The listing builds one solid part. Answer for the finished solid, in the listing's coordinates (mm). A direction names the side the tool comes from. Give positions to 0.01 mm unless a question says otherwise; leave off trailing zeros. Write each loop counter-clockwise with the first axis right and the second up, starting at its lowest first coordinate (ties: lowest second). Pieces come first, ordered by that corner, then holes. Notation, with made-up numbers: (-24.5, 2) - (-8.5, 2) arc R19 cw to (-8.5, 32) - close; hole circle Ø6 at (87, 80.5). An arc over 180 degrees is marked (long way). Answer as CSV lines item,"result". Start each with the question number.
(1) Each of these flat-tipped pins is pushed along its axis until it touches: pin 1 Ø5 at (x, z) = (-3, -5.5) entering from -Y; pin 2 Ø1.5 at (x, z) = (-34, -13.5) entering from +Y; pin 3 Ø4 at (x, z) = (-39, -30.5) entering from +Y. Where does it stop, or does it pass through?
(2) For a pull along Z with two mould halves and no side action, classify faces 1 (the face through (-33, 1, -7)), 2 (the face through (45, 10, 1)) as pulls with the +Z half, pulls with the -Z half, needs draft (parallel to the pull), parting line crosses it, or undercut.
(3) Find section C-C (x = -21). Write down the section's boundary in (y, z), then the cut area to 3 significant figures.
(4) Straight lines are drawn through the part: probe 1 along Z at (x, y) = (8.5, 11); probe 2 along X at (y, z) = (5.25, -25.5); probe 3 along X at (y, z) = (17, -26). For each, find the intervals that lie inside material, in ascending order.
(5) Find section B-B (z = 24). Write down the section's boundary in (x, y), then the cut area to 3 significant figures.
(6) For faces 3 (the face through (-28, 1, -7)), 4 (the face through (41, 5, -29)), 5 (the face through (33, 17, 35)), 6 (the face through (11.8, 4.5, 24)), 7 (the face through (-32.3, 1.5, 0)), determine the directions among +Z, -Z, +X, -X, +Y, -Y from which every point of the face is accessible in a straight line to the end or side of a thin tool.
(7) Find section D-D (z = 14.5). Write down the section's boundary in (x, y), then the cut area to 3 significant figures.
(8) Find section A-A (y = 16). Write down the section's boundary in (x, z), then the cut area to 3 significant figures.
from build123d import *

# Parameters (mm, degrees)
SKETCH_1_W                  = 90
SKETCH_1_H                  = 72
EXTRUDE_1_DEPTH             = 21
CUT_EXTRUDE_1_DEPTH         = 72
FILLET_1_R                  = 0.5
FILLET_2_R                  = 0.2
CUT_EXTRUDE_2_DEPTH         = 28
SKETCH_6_W                  = 5
SKETCH_6_H                  = 2
CUT_EXTRUDE_3_DEPTH         = 2.4
FILLET_3_R                  = 0.5
EXTRUDE_2_DEPTH             = 3.5
FILLET_4_R                  = 1
FILLET_5_R                  = 0.3
CHAMFER_1_SIZE              = 1
SKETCH_8_W                  = 2.9
SKETCH_8_H                  = 4
EXTRUDE_3_DEPTH             = 2.5
CHAMFER_2_SIZE              = 2
CHAMFER_2_SIZE2             = 1.400415076
FILLET_6_R                  = 0.2
FILLET_7_R                  = 0.3
FILLET_8_R                  = 0.2
SKETCH_9_W                  = 15.2
SKETCH_9_H                  = 5
CUT_EXTRUDE_4_DEPTH         = 36
SKETCH_10_W                 = 7.6
SKETCH_10_H                 = 5
CUT_EXTRUDE_5_DEPTH         = 4
CUT_EXTRUDE_6_DEPTH         = 72
SKETCH_12_W                 = 86
SKETCH_12_H                 = 68
CUT_EXTRUDE_7_DEPTH         = 14.5
SKETCH_13_W                 = 24
SKETCH_13_H                 = 16
CUT_EXTRUDE_8_DEPTH         = 5
MIRROR_4_COPY_1_SKETCH_W    = 24
MIRROR_4_COPY_1_SKETCH_H    = 16
MIRROR_4_COPY_1_DEPTH       = 5
EXTRUDE_4_DEPTH             = 7
MIRROR_6_COPY_1_DEPTH       = 7
SKETCH_15_W                 = 20
SKETCH_15_H                 = 2
EXTRUDE_5_DEPTH             = 2
SKETCH_17_W                 = 4
SKETCH_17_H                 = 2
EXTRUDE_6_DEPTH             = 1
CHAMFER_3_SIZE              = 1
CHAMFER_3_SIZE2             = 1.428148007
CHAMFER_3_OF_MIRROR_8_SIZE2 = 1.428148007
CHAMFER_3_OF_MIRROR_8_SIZE  = 1


with BuildPart() as part:
    # 草图1 → 凸台-拉伸1 (new body)
    with BuildSketch(Plane(origin=(0, 0, 0), x_dir=(1, 0, 0), z_dir=(0, 1, 0))):
        Rectangle(SKETCH_1_W, SKETCH_1_H)
    extrude(amount=EXTRUDE_1_DEPTH)

    # 草图4 → 切除-拉伸1 (cut)
    with BuildSketch(Plane.XY.offset(36)):
        Polygon((14.3, 0), (14.3, 1.5), (15.489963906, 2.965295015), (17.6, 3.5), (17.6, 5), (13.598917425, 4.003578801), (10, 5), (-17.6, 5), (-17.9, 0), align=None)
    extrude(amount=-CUT_EXTRUDE_1_DEPTH, mode=Mode.SUBTRACT)

    # 圆角1
    fillet_1_edges = [part.edges().sort_by_distance(p)[0] for p in [
        (17.6, 5, 0),
        (17.6, 3.5, 0),
    ]]
    fillet(fillet_1_edges, radius=FILLET_1_R)

    # 圆角2
    fillet_2_edges = [part.edges().sort_by_distance(p)[0] for p in [
        (14.3, 0, 0),
        (-17.9, 0, 0),
        (-17.6, 5, 0),
        (15.489963906, 2.965295015, 0),
        (14.3, 1.5, 0),
    ]]
    fillet(fillet_2_edges, radius=FILLET_2_R)

    # 草图5 → 切除-拉伸2 (cut)
    with BuildSketch(Plane.ZY.offset(45)):
        Polygon((5.6, 0), (5.6, 2.4), (7.6, 2.4), (7.6, 5), (-7.6, 5), (-7.6, 2.4), (-5.6, 2.4), (-5.6, 0), align=None)
    extrude(amount=-CUT_EXTRUDE_2_DEPTH, mode=Mode.SUBTRACT)

    # 草图6 → 切除-拉伸3 (cut)
    with BuildSketch(Plane.XZ):
        with Locations((-30.5, 6.6)):
            Rectangle(SKETCH_6_W, SKETCH_6_H)
    cut_extrude_3 = extrude(amount=-CUT_EXTRUDE_3_DEPTH, mode=Mode.SUBTRACT)

    # 镜向1: 切除-拉伸3 across plane
    add(cut_extrude_3.mirror(Plane(origin=(0, 0, 0), x_dir=(1, 0, 0), z_dir=(0, 0, -1))), mode=Mode.SUBTRACT)

    # 圆角3
    fillet_3_edges = [part.edges().sort_by_distance(p)[0] for p in [
        (-31.205820162, 5, -7.6),
        (-31.205820162, 5, 7.6),
    ]]
    fillet(fillet_3_edges, radius=FILLET_3_R)

    # 草图7 → 凸台-拉伸2 (add)
    with BuildSketch(Plane.XZ.offset(-5)):
        Polygon((-33, 3.2), (-33, -3.2), (-28, -3.2), (-32, -1), (-32, 1), (-28, 3.2), align=None)
    extrude(amount=EXTRUDE_2_DEPTH)

    # 圆角4
    fillet_4_edges = [part.edges().sort_by_distance(p)[0] for p in [
        (-32, 3.25, -1),
        (-32, 3.25, 1),
    ]]
    fillet(fillet_4_edges, radius=FILLET_4_R)

    # 圆角5
    fillet_5_edges = [part.edges().sort_by_distance(p)[0] for p in [
        (-28, 3.25, 3.2),
        (-28, 3.25, -3.2),
    ]]
    fillet(fillet_5_edges, radius=FILLET_5_R)

    # 倒角1
    chamfer_1_edges = [part.edges().sort_by_distance(p)[0] for p in [
        (-33, 3.25, 3.2),
        (-33, 3.25, -3.2),
    ]]
    chamfer(chamfer_1_edges, length=CHAMFER_1_SIZE)

    # 草图8 → 凸台-拉伸3 (add)
    with BuildSketch(Plane.XZ.offset(-5)):
        with Locations((-35.91, 0)):
            Rectangle(SKETCH_8_W, SKETCH_8_H)
    extrude(amount=EXTRUDE_3_DEPTH)

    # 倒角2
    chamfer_2_edges = [part.edges().sort_by_distance(p)[0] for p in [
        (-34.46, 2.5, 0),
    ]]
    chamfer_2_side = [part.faces().sort_by_distance(p)[0] for p in [
        (-35.91, 2.5, 0),
    ]]
    chamfer(chamfer_2_edges, length=CHAMFER_2_SIZE, length2=CHAMFER_2_SIZE2, reference=chamfer_2_side[0])

    # 圆角6
    fillet_6_edges = [part.edges().sort_by_distance(p)[0] for p in [
        (-37.36, 5, 0),
        (-37.36, 3.75, 2),
        (-35.91, 5, -2),
        (-37.36, 3.75, -2),
        (-34.46, 5, 0),
        (-35.91, 5, 2),
        (-37.36, 2.5, 0),
        (-36.91, 2.5, -2),
        (-34.46, 4.450207538, -2),
        (-35.46, 3.200207538, -2),
    ]]
    fillet(fillet_6_edges, radius=FILLET_6_R)

    # 圆角7
    # the kernel refuses this fillet: 0.3 mm, written as the material it takes off along each edge
    with BuildSketch(Plane(origin=(-36.554589637, 2.8, -2), x_dir=(0.5735764363510475, -0.8191520442889909, 0), z_dir=(0.8191520442889909, 0.5735764363510475, 0))) as fillet_7_piece_1:
        with BuildLine():
            CenterArc((0.1, -0.2), 0.2, 0, 90)
            Line((0.3, -0.2), (0.3, 0))
            Line((0.3, 0), (0.1, 0))
        make_face()
    revolve(axis=Axis((-36.554589637, 2.8, -2), (0, 0, -1)), revolution_arc=35, mode=Mode.SUBTRACT)
    with BuildSketch(Plane(origin=(-36.46, 2.5, 2.236474092), x_dir=(0.8191520442890007, 0.5735764363510335, 0), z_dir=(0, 0, -1))) as fillet_7_piece_2:
        with BuildLine():
            CenterArc((FILLET_7_R * 0.315298788879, -FILLET_7_R), FILLET_7_R, 90, 35)
            Line((-FILLET_7_R * 0.258277647472, -FILLET_7_R * 0.180847955711), (0, 0))
            Line((0, 0), (FILLET_7_R * 0.315298788879, 0))
        make_face()
    extrude(amount=4.236474092, mode=Mode.SUBTRACT)

    # 圆角8
    fillet_8_edges = [part.edges().sort_by_distance(p)[0] for p in [
        (-34.46, 3.900415076, 0.1),
        (-34.522857251, 3.93313649, -1.945574265),
    ]]
    fillet(fillet_8_edges, radius=FILLET_8_R)

    # 草图9 → 切除-拉伸4 (cut)
    with BuildSketch(Plane(origin=(45, 0, 0), x_dir=(0, 0, -1), z_dir=(1, 0, 0))):
        with Locations((0, 2.5)):
            Rectangle(SKETCH_9_W, SKETCH_9_H)
    extrude(amount=-CUT_EXTRUDE_4_DEPTH, mode=Mode.SUBTRACT)

    # 草图10 → 切除-拉伸5 (cut)
    with BuildSketch(Plane(origin=(0, 0, 7.6), x_dir=(-1, 0, 0), z_dir=(0, 0, -1))):
        with Locations((-13.8, 2.5)):
            Rectangle(SKETCH_10_W, SKETCH_10_H)
    cut_extrude_5 = extrude(amount=-CUT_EXTRUDE_5_DEPTH, mode=Mode.SUBTRACT)

    # 镜向2: 切除-拉伸5 across plane
    add(cut_extrude_5.mirror(Plane(origin=(0, 0, 0), x_dir=(1, 0, 0), z_dir=(0, 0, -1))), mode=Mode.SUBTRACT)

    # 草图11 → 切除-拉伸6 (cut)
    with BuildSketch(Plane.XY.offset(36)):
        Polygon((-37, 21), (37, 21), (28.3, 12.3), (-28.3, 12.3), align=None)
    extrude(amount=-CUT_EXTRUDE_6_DEPTH, mode=Mode.SUBTRACT)

    # 草图12 → 切除-拉伸7 (cut)
    with BuildSketch(Plane(origin=(0, 21, 0), x_dir=(1, 0, 0), z_dir=(0, 1, 0))):
        Rectangle(SKETCH_12_W, SKETCH_12_H)
    extrude(amount=-CUT_EXTRUDE_7_DEPTH, mode=Mode.SUBTRACT)

    # 草图13 → 切除-拉伸8 (cut)
    with BuildSketch(Plane(origin=(0, 6.5, 0), x_dir=(1, 0, 0), z_dir=(0, 1, 0))):
        with Locations((31, -26)):
            Rectangle(SKETCH_13_W, SKETCH_13_H)
    cut_extrude_8 = extrude(amount=-CUT_EXTRUDE_8_DEPTH, mode=Mode.SUBTRACT)

    # 镜向3: 切除-拉伸8 across plane
    add(cut_extrude_8.mirror(Plane(origin=(0, 0, 0), x_dir=(1, 0, 0), z_dir=(0, 0, -1))), mode=Mode.SUBTRACT)

    # 镜向4: 切除-拉伸8 across plane
    add(cut_extrude_8.mirror(Plane.ZY), mode=Mode.SUBTRACT)

    # 镜向4 copy 1 sketch → 镜向4 copy 1 (cut)
    with BuildSketch(Plane(origin=(0, 6.5, 0), x_dir=(-1, 0, 0), z_dir=(0, 1, 0))):
        with Locations((31, -26)):
            Rectangle(MIRROR_4_COPY_1_SKETCH_W, MIRROR_4_COPY_1_SKETCH_H)
    extrude(amount=-MIRROR_4_COPY_1_DEPTH, mode=Mode.SUBTRACT)

    # 草图14 → 凸台-拉伸4 (add)
    with BuildSketch(Plane(origin=(0, 1.5, 0), x_dir=(1, 0, 0), z_dir=(0, 1, 0))):
        Polygon((35, -34), (43, -34), (43, -26), (41, -26), (41, -32), (35, -32), align=None)
    extrude_4 = extrude(amount=EXTRUDE_4_DEPTH)

    # 镜向5: 凸台-拉伸4 across plane
    add(extrude_4.mirror(Plane(origin=(0, 0, 0), x_dir=(1, 0, 0), z_dir=(0, 0, -1))))

    # 镜向6: 凸台-拉伸4 across plane
    add(extrude_4.mirror(Plane.ZY))

    # 镜向6 copy 1 sketch → 镜向6 copy 1 (add)
    with BuildSketch(Plane(origin=(0, 1.5, 0), x_dir=(-1, 0, 0), z_dir=(0, 1, 0))):
        Polygon((35, -34), (43, -34), (43, -26), (41, -26), (41, -32), (35, -32), align=None)
    extrude(amount=MIRROR_6_COPY_1_DEPTH)

    # 草图15 → 凸台-拉伸5 (add)
    with BuildSketch(Plane(origin=(0, 6.5, 0), x_dir=(1, 0, 0), z_dir=(0, 1, 0))):
        with Locations((0, 33)):
            Rectangle(SKETCH_15_W, SKETCH_15_H)
    extrude_5 = extrude(amount=EXTRUDE_5_DEPTH)

    # 镜向7: 凸台-拉伸5 across plane
    add(extrude_5.mirror(Plane(origin=(0, 0, 0), x_dir=(1, 0, 0), z_dir=(0, 0, -1))))

    # 草图17 → 凸台-拉伸6 (add)
    with BuildSketch(Plane.XY.offset(-34)):
        with Locations((0, 11.3)):
            Rectangle(SKETCH_17_W, SKETCH_17_H)
    extrude_6 = extrude(amount=EXTRUDE_6_DEPTH)

    # 倒角3
    chamfer_3_edges = [part.edges().sort_by_distance(p)[0] for p in [
        (0, 12.3, -33),
    ]]
    chamfer_3_side = [part.faces().sort_by_distance(p)[0] for p in [
        (0, 12.3, -34.948805461),
    ]]
    chamfer(chamfer_3_edges, length=CHAMFER_3_SIZE, length2=CHAMFER_3_SIZE2, reference=chamfer_3_side[0])

    # 镜向8: 凸台-拉伸6 across plane
    add(extrude_6.mirror(Plane(origin=(0, 0, 0), x_dir=(1, 0, 0), z_dir=(0, 0, -1))))

    # 倒角3 of 镜向8
    chamfer_3_of_mirror_8_edges = [part.edges().sort_by_distance(p)[0] for p in [
        (0, 12.3, 33),
    ]]
    chamfer(chamfer_3_of_mirror_8_edges, length=CHAMFER_3_OF_MIRROR_8_SIZE, length2=CHAMFER_3_OF_MIRROR_8_SIZE2)


solid = part.part
Result set:
1,pin 1,"y = 5"
1,pin 2,"y = 6.5"
1,pin 3,"y = 8.5"
2,face 1,"undercut"
2,face 2,"needs draft"
3,outline,"(0, -36) - (12.3, -36) - (12.3, -34) - (1.5, -34) - (1.5, -18) - (6.5, -18) - (6.5, 18) - (1.5, 18) - (1.5, 34) - (12.3, 34) - (12.3, 36) - (0, 36) - (0, 5.6) - (2.4, 5.6) - (2.4, 7.6) - (4.5, 7.6) arc R0.5 cw to (5, 7.1) - (5, -7.1) arc R0.5 cw to (4.5, -7.6) - (2.4, -7.6) - (2.4, -5.6) - (0, -5.6) - close"
3,area,"265 mm^2"
4,probe 1,"-36 to -34, 34 to 36"
4,probe 2,"-45 to -43, -19 to 19, 43 to 45"
4,probe 3,"-45 to -43, 43 to 45"
5,outline,"(-45, 0) - (-18.09, 0) arc R0.2 ccw to (-17.89, 0.19) - (-17.61, 4.81) arc R0.2 cw to (-17.41, 5) - (10, 5) - (13.6, 4) - (16.98, 4.85) arc R0.5 cw to (17.6, 4.36) - (17.6, 3.89) arc R0.5 cw to (17.22, 3.4) - (15.55, 2.98) arc R0.2 ccw to (15.45, 2.91) - (14.34, 1.56) arc R0.2 ccw to (14.3, 1.43) - (14.3, 0.2) arc R0.2 ccw to (14.5, 0) - (45, 0) - (45, 21) - (43, 21) - (43, 1.5) - (19, 1.5) - (19, 6.5) - (-19, 6.5) - (-19, 1.5) - (-43, 1.5) - (-43, 21) - (-45, 21) - close"
5,area,"240 mm^2"
6,face 3,"-Y"
6,face 4,"+Y"
6,face 5,"+Z, -Z, +Y"
6,face 6,"+Z, -Z, -Y"
6,face 7,"+X, -X, -Y"
7,outline,"(-45, 0) - (-18.09, 0) arc R0.2 ccw to (-17.89, 0.19) - (-17.61, 4.81) arc R0.2 cw to (-17.41, 5) - (10, 5) - (13.6, 4) - (16.98, 4.85) arc R0.5 cw to (17.6, 4.36) - (17.6, 3.89) arc R0.5 cw to (17.22, 3.4) - (15.55, 2.98) arc R0.2 ccw to (15.45, 2.91) - (14.34, 1.56) arc R0.2 ccw to (14.3, 1.43) - (14.3, 0.2) arc R0.2 ccw to (14.5, 0) - (45, 0) - (45, 21) - (43, 21) - (43, 6.5) - (-43, 6.5) - (-43, 21) - (-45, 21) - close"
7,area,"480 mm^2"
8,outline,"(-45, -36) - (-32, -36) - (-32, -34) - (-43, -34) - (-43, 34) - (-32, 34) - (-32, 36) - (-45, 36) - close; (32, -36) - (45, -36) - (45, 36) - (32, 36) - (32, 34) - (43, 34) - (43, -34) - (32, -34) - close"
8,area,"376 mm^2"
